Design review of the part built by this model. Coordinates are the model's own, in mm. Face numbers are marked on the shaded views. A direction names the side the tool comes from. Coordinates: 2 decimals unless noted, no trailing zeros. Loops run counter-clockwise (first coordinate to the right, second up) from the corner with the lowest first, then second, coordinate; pieces in that order, holes last. Notation, with made-up numbers: (11, -7) - (23, -7) arc R9 ccw to (23, 6) - close; hole circle Ø11 at (-10.5, 23). An arc over 180 degrees is marked (long way). Answer in a Markdown table with one row per item. Add a question column.
(1) We need section B-B, the plane y = 3.5. Write out the cut boundary in (x, z).
(2) Clearance check with flat-ended pins moving along their axes: pin 1 (0.9 mm diameter, centred on x = -19.5, y = 0.5, fed in from +Z); pin 2 (9.5 mm diameter, centred on x = 20, y = -4, fed in from +Z). State where each tip first meets the part, or that it passes through.
(3) For the marked faces 3 and 4, list the 3-axis set-ups (+Z, -Z, +X, -X, +Y, -Y) from which the entire face can be reached by the end or side of a thin tool; tool diameter is ignored.
(4) The part is to be moulded in two halves that separate along X. For the marked faces 1 and 2, say which applies: released by +X, released by -X, zero draft, split by the parting line, or undercut.
(5) We need section A-A, the plane x = 28. Write out the cut boundary in (y, z), plus the area to 3 significant figures.
(6) To check wall thickness, follow L1, parallel to Y at x = 38, z = 2.95; L2, parallel to Y at x = 8.5, z = 2.65; L3, parallel to X at y = 0, z = 1.9. State the ranges of each line that lie inside material, in increasing order. Write a range as [from, to].
from build123d import *

# Parameters (mm, degrees)
F0_W      = 100
F0_H      = 40
F1_DEPTH  = 4
F2_W      = 75
F2_H      = 20
F3_DEPTH  = 2
F5_R      = 2.5
F6_DEPTH  = 9
F7_DEPTH  = 40.001
F9_SIZE   = 0.6
F8_W      = 0.8
F8_H      = 20
F10_DEPTH = 0.6


with BuildPart() as f1:
    # F0 (on Top) → F1 (new body)
    with BuildSketch(Plane.XY):
        Rectangle(F0_W, F0_H)
    extrude(amount=F1_DEPTH)

    # F2 (on face) → F3 (cut)
    with BuildSketch(Plane.XY.offset(4)):
        Rectangle(F2_W, F2_H)
    extrude(amount=-F3_DEPTH, mode=Mode.SUBTRACT)

    # F5 (on Front) → F6 (cut, symmetric)
    with BuildSketch(Plane.XZ):
        with Locations((39.1, 4)):
            Circle(F5_R)
    extrude(amount=F6_DEPTH, both=True, mode=Mode.SUBTRACT)

    # F4 (on face) → F7 (cut, through all)
    with BuildSketch(Plane.XZ.offset(20)):
        with BuildLine():
            ThreePointArc((-33.8, 4), (-33, 3.2), (-32.2, 4))
            Line((-32.2, 4), (-33.8, 4))
        make_face()
        with BuildLine():
            Line((-23.2, 4), (-24.8, 4))
            ThreePointArc((-24.8, 4), (-24, 3.2), (-23.2, 4))
        make_face()
        with BuildLine():
            Line((-14.2, 4), (-15.8, 4))
            ThreePointArc((-15.8, 4), (-15, 3.2), (-14.2, 4))
        make_face()
        with BuildLine():
            Line((39.9, 4), (38.3, 4))
            ThreePointArc((38.3, 4), (39.1, 3.2), (39.9, 4))
        make_face()
    extrude(amount=-F7_DEPTH, mode=Mode.SUBTRACT)

    # F9
    f9_edges = [f1.edges().sort_by_distance(p)[0] for p in [
        (0, 10, 2),
        (0, -10, 2),
    ]]
    chamfer(f9_edges, length=F9_SIZE)

    # F8 (on face) → F10 (join)
    with BuildSketch(Plane.XY.offset(2)):
        with Locations((-28.5, 0)):
            Rectangle(F8_W, F8_H)
        with Locations((-19.5, 0)):
            Rectangle(F8_W, F8_H)
        with Locations((-10.5, 0)):
            Rectangle(F8_W, F8_H)
    extrude(amount=F10_DEPTH)


solid = f1.part
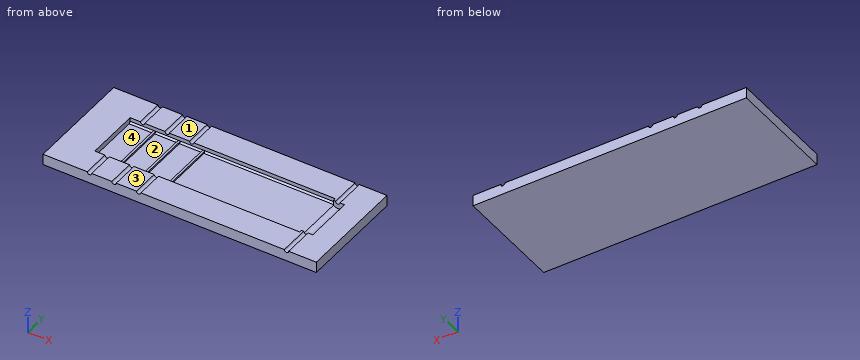
Responses:
| question | item | result |
|---|---|---|
| 1 | outline | (-50, 0) - (50, 0) - (50, 4) - (41.6, 4) arc R2.5 cw to (37.5, 2.08) - (37.5, 2) - (-10.1, 2) - (-10.1, 2.6) - (-10.9, 2.6) - (-10.9, 2) - (-19.1, 2) - (-19.1, 2.6) - (-19.9, 2.6) - (-19.9, 2) - (-28.1, 2) - (-28.1, 2.6) - (-28.9, 2.6) - (-28.9, 2) - (-37.5, 2) - (-37.5, 4) - (-50, 4) - close |
| 2 | pin 1 | stops at z = 2.6 |
| 2 | pin 2 | stops at z = 2 |
| 3 | face 3 | +Z, +X, -X, +Y, -Y |
| 3 | face 4 | +Z |
| 4 | face 1 | zero draft |
| 4 | face 2 | undercut |
| 5 | outline | (-20, 0) - (20, 0) - (20, 4) - (10, 4) - (10, 2.6) - (9.4, 2) - (-9.4, 2) - (-10, 2.6) - (-10, 4) - (-20, 4) - close |
| 5 | area | 120 mm2 |
| 6 | L1 | y = [-20, -9], [9, 20] |
| 6 | L2 | y = [-20, -10], [10, 20] |
| 6 | L3 | x = [-50, 37.74], [40.46, 50] |
